```python
from build123d import *

# Parameters (mm, degrees)
SKETCH_R     = 100
SKETCH_R_2   = 80
PAD_DEPTH    = 40
THICKNESS_T  = -5
PAD001_DEPTH = 40
POCKET_DEPTH = 35


with BuildPart() as part:
    # Sketch → Pad (new body)
    with BuildSketch(Plane.XZ):
        Circle(SKETCH_R)
        Circle(SKETCH_R_2, mode=Mode.SUBTRACT)
    extrude(amount=PAD_DEPTH)

    # Thickness
    thickness_openings = [part.faces().sort_by_distance(p)[0] for p in [
        (-97.171573, 0, 0),
    ]]
    offset(amount=THICKNESS_T, openings=thickness_openings)

    # Sketch001 → Pad001 (join)
    with BuildSketch(Plane.XZ):
        with BuildLine():
            Line((-60, -105), (-60, -115))
            ThreePointArc((-60, -115), (-57.071068, -122.071068), (-50, -125))
            Line((-50, -125), (50, -125))
            ThreePointArc((50, -125), (57.071068, -122.071068), (60, -115))
            Line((60, -115), (60, -105))
            ThreePointArc((60, -105), (57.071068, -97.928932), (50, -95))
            Line((50, -95), (-50, -95))
            ThreePointArc((-50, -95), (-57.071068, -97.928932), (-60, -105))
        make_face()
    extrude(amount=PAD001_DEPTH)

    # Sketch002 (on Face11 of Pad001) → Pocket (cut)
    with BuildSketch(Plane.XZ.offset(40)):
        with BuildLine():
            Line((-55, -105), (-55, -115))
            ThreePointArc((-55, -115), (-53.535534, -118.535534), (-50, -120))
            Line((-50, -120), (50, -120))
            ThreePointArc((50, -120), (53.535534, -118.535534), (55, -115))
            Line((55, -115), (55, -105))
            ThreePointArc((55, -105), (53.535534, -101.464466), (50, -100))
            Line((50, -100), (-50, -100))
            ThreePointArc((-50, -100), (-53.535534, -101.464466), (-55, -105))
        make_face()
    extrude(amount=-POCKET_DEPTH, mode=Mode.SUBTRACT)


solid = part.part
```
Input: part model. Units: mm. Frame: model coordinates. A direction names the side the tool comes from. Give positions to 0.01 mm unless a question says otherwise; leave off trailing zeros. Order: outer loops, then holes, each group sorted by start corner. A loop starts at its lowest first (then second) coordinate and runs counter-clockwise, first axis right, second up.
1. Material intervals for L1, parallel to Z at x = 0, y = -7; L2, parallel to Z at x = 12.5, y = -23; L3, parallel to X at y = -25, z = 58.5, sorted ascending.
Derived:
L1: z = -125 to -120, -100 to -95, -85 to -80, 80 to 85, 95 to 100
L2: z = -125 to -120, -100 to -94.17, -84.08 to -79.02, 79.02 to 84.08, 94.17 to 99.22
L3: x = -81.1 to -74.85, -61.67 to -54.57, 54.57 to 61.67, 74.85 to 81.1
2. Pin query (flat end, axial travel): pin 1 (8 mm diameter, centred on y = -25, z = -110.5, fed in from +X); pin 2 (2 mm diameter, centred on y = -14.5, z = 59.5, fed in from +X); pin 3 (11 mm diameter, centred on y = -22, z = -111, fed in from -X). Return the tip coordinate at first contact, or that it passes through.
Derived:
pin 1: stops at x = 60
pin 2: stops at x = 81.1
pin 3: stops at x = -60
3. Reachability of faces 4 (the cylindrical face through (-67.453, -17.255, -51.721)), 5 (the cylindrical face through (-53, -23, -101)), 6 (the cylindrical face through (-56.99, -19.72, -97.85)), 7 (the flat face through (60, -20, -110)), 8 (the cylindrical face through (-17.34, -19.72, -78.1)) from +Z, -Z, +X, -X, +Y, -Y: full face, straight path, thin tool, end or side. Return the list, or none.
Derived:
face 4: +Y
face 5: -Y
face 6: -X, +Y, -Y
face 7: -Z, +X, +Y, -Y
face 8: +Y, -Y
4. Section B-B on x = 0. Return the cut outline in (y, z).
Derived:
outline: (-40, -125) - (0, -125) - (0, -95) - (-35, -95) - (-35, -85) - (0, -85) - (0, -80) - (-40, -80) - (-40, -100) - (-5, -100) - (-5, -120) - (-40, -120) - close; (-40, 80) - (0, 80) - (0, 85) - (-35, 85) - (-35, 95) - (0, 95) - (0, 100) - (-40, 100) - close
5. Section C-C on y = -17. Return the cut outline in (x, z).
Derived:
outline: circle Ø170 at (0, 0); (-60, -115) arc R10 ccw to (-50, -125) - (50, -125) arc R10 ccw to (60, -115) - (60, -105) arc R10 ccw to (50, -95) - (31.22, -95) arc R100 ccw (long way) to (-31.22, -95) - (-50, -95) arc R10 ccw to (-60, -105) - close; hole circle Ø190 at (0, 0); hole circle Ø160 at (0, 0); hole (-55, -115) arc R5 ccw to (-50, -120) - (50, -120) arc R5 ccw to (55, -115) - (55, -105) arc R5 ccw to (50, -100) - (-50, -100) arc R5 ccw to (-55, -105) - close
6. Section D-D on z = -27.5. Return the cut outline in (x, y).
Derived:
outline: (-96.14, -40) - (-75.12, -40) - (-75.12, 0) - (-80.43, 0) - (-80.43, -35) - (-90.93, -35) - (-90.93, 0) - (-96.14, 0) - close; (75.12, -40) - (96.14, -40) - (96.14, 0) - (90.93, 0) - (90.93, -35) - (80.43, -35) - (80.43, 0) - (75.12, 0) - close
7. Mould query, pull axis X, two halves, no side actions, for faces 1 (the flat face through (-1, -20, -125)), 2 (the cylindrical face through (57.15, -19.72, -98.01)), 3 (the flat face through (-1, -5, -110)). Classes: released by +X, released by -X, zero draft, split by the parting line, or undercut.
Derived:
face 1: zero draft
face 2: released by +X
face 3: undercut
8. Section A-A on z = 0. Return the cut outline in (x, y), and give its area (3 significant figures).
Derived:
outline: (-100, -40) - (-80, -40) - (-80, 0) - (-85, 0) - (-85, -35) - (-95, -35) - (-95, 0) - (-100, 0) - close; (80, -40) - (100, -40) - (100, 0) - (95, 0) - (95, -35) - (85, -35) - (85, 0) - (80, 0) - close
area: 900 mm2
